```python
from build123d import *

# Parameters (mm, degrees)
BOSS_EXTRUDE1_DEPTH     = 20
FILLET1_R               = 7.62
SKETCH2_W               = 14.64163524
SKETCH2_H               = 15
CUT_EXTRUDE3_DEPTH      = 4.607313514
CUT_EXTRUDE3_DEPTH_BACK = 3
SKETCH3_W               = 1.5
SKETCH3_H               = 1
CUT_EXTRUDE4_DEPTH      = 22.118365096


with BuildPart() as part:
    # Sketch1 → Boss-Extrude1 (new body)
    with BuildSketch(Plane.XY):
        with BuildLine():
            Line((-21.118365096, 5.5), (-17.118365096, 8.408769901))
            Line((-17.118365096, 8.408769901), (-10.829358836, 12.039729358))
            Line((-10.829358836, 12.039729358), (-3.209358836, 12.039729358))
            Line((-3.209358836, 12.039729358), (1.290641164, 7.539729358))
            Line((1.290641164, 7.539729358), (-0.508988662, 7.539729358))
            ThreePointArc((-0.508988662, 7.539729358), (-2.01251766, 7.308314112), (-3.376870844, 6.635489579))
            Line((-3.376870844, 6.635489579), (-4.998518024, 5.5))
            Line((-4.998518024, 5.5), (-21.118365096, 5.5))
        make_face()
    extrude(amount=-BOSS_EXTRUDE1_DEPTH)

    # Fillet1
    fillet1_edges = [part.edges().sort_by_distance(p)[0] for p in [
        (-3.209358836, 12.039729358, -10),
        (-10.829358836, 12.039729358, -10),
    ]]
    fillet(fillet1_edges, radius=FILLET1_R)

    # Sketch2 → Cut-Extrude3 (cut, two sides)
    with BuildSketch(Plane(origin=(-4.228616794, 6.039090645, 0), x_dir=(0.819152044, 0.573576436, 0), z_dir=(0.573576436, -0.819152044, 0))) as cut_extrude3_sk:
        with Locations((7.360607431, -10)):
            Rectangle(SKETCH2_W, SKETCH2_H)
    extrude(amount=CUT_EXTRUDE3_DEPTH, mode=Mode.SUBTRACT)
    extrude(cut_extrude3_sk.sketch, amount=-CUT_EXTRUDE3_DEPTH_BACK, mode=Mode.SUBTRACT)

    # Sketch3 → Cut-Extrude4 (cut, through all)
    with BuildSketch(Plane(origin=(0, 0, 0), x_dir=(0, 0, -1), z_dir=(1, 0, 0))):
        with Locations((10, 6)):
            Rectangle(SKETCH3_W, SKETCH3_H)
    extrude(amount=-CUT_EXTRUDE4_DEPTH, mode=Mode.SUBTRACT)


solid = part.part
```
For this review, take the finished solid that the model builds, in its own axes (mm). A direction names the side the tool comes from. Coordinates: 2 decimals unless noted, no trailing zeros. Write each loop counter-clockwise with the first axis right and the second up, starting at its lowest first coordinate (ties: lowest second). Pieces come first, ordered by that corner, then holes.
(1) Add section B-B on x = -13.25. Give the boundary of the cut face in (y, z), then the cut area to 3 significant figures.
(2) For pin 1 Ø0.8 at (x, z) = (-11.5, -10.5) entering from -Y; pin 2 Ø2 at (x, z) = (0.5, -19.5) entering from -Y; pin 3 Ø12 at (x, z) = (-17, -6) entering from +Y; pin 4 Ø4 at (x, z) = (-18.5, -16.5) entering from +Y, all flat-tipped, find the tip position at first contact; note any pin that passes through.
(3) Add section C-C on z = -14.75. Give the boundary of the cut face in (x, y), then the cut area to 3 significant figures.
(4) Add section A-A on z = -10.25. Give the boundary of the cut face in (x, y), then the cut area to 3 significant figures.
(5) The part is to be moulded in two halves that separate along Y. For faces 1 (the face through (-10.79, 11.77, -10.14)), 2 (the face through (-1.992, 7.315, -18.732)), 3 (the face through (-3, 8, -17.5)), say which applies: +Y half, -Y half, draft (parallel to the pull), parting line (faces both ways), or undercut.
(6) Wall thickness on probe 1 along Z at (x, y) = (-2, 9); probe 2 along Z at (x, y) = (-18.5, 6.25); probe 3 along Y at (x, z) = (-19.75, -16.25): over which ranges is each line inside the solid? List them lowest first.
(7) Add section D-D on y = 11.5. Give the boundary of the cut face in (x, z).
(8) Tool access review of faces 4 (the face through (-19.15, 6.93, -9.86)), 5 (the face through (-13, 6, -10.75)), 6 (the face through (0, 7.54, -19)), 7 (the face through (-4.2, 9.72, -9.9)): name each direction out of +Z, -Z, +X, -X, +Y, -Y from which nothing blocks a thin tool from reaching the whole face with its end or side.
Answer sheet:
1. outline: (5.5, -20) - (10.64, -20) - (10.64, 0) - (5.5, 0) - (5.5, -9.25) - (6.5, -9.25) - (6.5, -10.75) - (5.5, -10.75) - close
1. area: 101 mm2
2. pin 1: stops at y = 5.5
2. pin 2: stops at y = 7.54
2. pin 3: stops at y = 11.71
2. pin 4: stops at y = 8.77
3. outline: (-21.12, 5.5) - (-5, 5.5) - (-4.2, 6.06) - (-5.92, 8.52) - (-2.44, 10.95) arc R7.62 ccw to (-6.37, 12.04) - (-8.79, 12.04) arc R7.62 ccw to (-12.6, 11.02) - (-17.12, 8.41) - close
3. area: 76.8 mm2
4. outline: (-19.74, 6.5) - (-4.5, 6.5) - (-5.92, 8.52) - (-2.44, 10.95) arc R7.62 ccw to (-6.37, 12.04) - (-8.79, 12.04) arc R7.62 ccw to (-12.6, 11.02) - (-17.12, 8.41) - close
4. area: 60.8 mm2
5. face 1: +Y half
5. face 2: -Y half
5. face 3: undercut
6. probe 1: z = -20 to -17.5, -2.5 to 0
6. probe 2: z = -20 to -10.75, -9.25 to 0
6. probe 3: y = 5.5 to 6.5
7. outline: (-11.6, -20) - (-3.55, -20) - (-3.55, 0) - (-11.6, 0) - close
8. face 4: +Z, -Z, -X, +Y
8. face 5: +X, -X, -Y
8. face 6: +Z, -Z, +X, -Y
8. face 7: +X
